Can you work these out from the model? Positions are in its coordinate system, mm. Face numbers are marked on the shaded views. Round coordinates to 2 decimals unless told otherwise and drop trailing zeros. Write each loop counter-clockwise with the first axis right and the second up, starting at its lowest first coordinate (ties: lowest second). Pieces come first, ordered by that corner, then holes. Notation, with made-up numbers: (42, -30) - (84, -30) arc R21 cw to (84, 1) - close; hole circle Ø2 at (-26.5, 62). An arc over 180 degrees is marked (long way). One line per item, written item: value. Start each with the question number.
(1) Thinking about a two-plate mould opening in Y: for the marked faces 1, 2 and 3, which applies, +Y half, -Y half, draft (parallel to the pull), parting line (faces both ways), or undercut?
(2) I want a section at D-D on x = 20. List the corners of the cut face in (y, z) for me.
(3) I want a section at C-C on y = -6. List the corners of the cut face in (x, z) for me.
(4) I'm going to push flat-ended pins straight in: pin 1 Ø1.1 at (y, z) = (-3, 8.5) entering from +X; pin 2 Ø0.6 at (x, y) = (26, -6.5) entering from -Z; pin 3 Ø1.1 at (x, y) = (13.5, 2.5) entering from -Z. Where does each tip first touch, or does it pass through?
(5) If I drill on L1, parallel to Y at x = 25.5, z = 19; L2, parallel to Y at x = 16.5, z = 11.75; L3, parallel to Y at x = 34, z = 23, over which ranges is the centre line in solid material (lowest first)? Write a range as from..to.
(6) I want a section at B-B on z = 17. List the corners of the cut face in (x, y) for me, plus the area to 3 significant figures.
(7) I want a section at A-A on z = 20.5. List the corners of the cut face in (x, y) for me.
from build123d import *

# Parameters (mm, degrees)
SKETCH1_W           = 3
SKETCH1_H           = 21.71695
SKETCH1_W_2         = 2.8
SKETCH1_H_2         = 4
SKETCH1_W_3         = 0.2
BOSS_EXTRUDE3_DEPTH = 1.36
BOSS_EXTRUDE4_START = -1.36
SKETCH1_7_W         = 3
SKETCH1_7_H         = 21.71695
SKETCH1_7_W_2       = 2.8
SKETCH1_7_H_2       = 4
SKETCH1_7_W_3       = 0.2
BOSS_EXTRUDE4_DEPTH = 2.2
BOSS_EXTRUDE5_START = -3.56
SKETCH1_8_W         = 3
SKETCH1_8_H         = 21.71695
BOSS_EXTRUDE5_DEPTH = 1.7
BOSS_EXTRUDE6_START = -5.26
SKETCH1_9_W         = 3
SKETCH1_9_H         = 21.71695
SKETCH1_9_W_2       = 2.8
SKETCH1_9_H_2       = 4
SKETCH1_9_W_3       = 0.2
BOSS_EXTRUDE6_DEPTH = 2
SKETCH2_W           = 43.56375
SKETCH2_H           = 3
BOSS_EXTRUDE7_DEPTH = 1.8
BOSS_EXTRUDE8_START = 1.8
SKETCH2_3_W         = 43.56375
SKETCH2_3_H         = 3
BOSS_EXTRUDE8_DEPTH = 1.8


with BuildPart() as part:
    # Sketch1 → Boss-Extrude3 (new body)
    with BuildSketch(Plane(origin=(0, 0, 0), x_dir=(1, 0, 0), z_dir=(0, 1, 0))):
        Polygon((2.8, -21.51695), (-0.2, -21.51695), (-3.2, -21.51695), (-3.2, -24.51695), (40.36375, -24.51695), (40.36375, -21.51695), align=None)
        with Locations((-1.7, -10.658475)):
            Rectangle(SKETCH1_W, SKETCH1_H)
        Polygon((0, 0), (0, -21.31695), (2.8, -21.31695), (2.8, -18.51695), (2.8, 0), align=None)
        Polygon((40.16375, 0), (2.8, 0), (2.8, -18.51695), (37.36375, -18.51695), (37.36375, -14.51695), (40.16375, -14.51695), align=None)
        Polygon((2.8, -18.51695), (2.8, -21.31695), (40.16375, -21.31695), (40.16375, -18.51695), (37.36375, -18.51695), align=None)
        with Locations((38.76375, -16.51695)):
            Rectangle(SKETCH1_W_2, SKETCH1_H_2)
        Polygon((43.36375, -14.51695), (40.36375, -14.51695), (40.36375, -18.51695), (40.36375, -21.51695), (40.36375, -24.51695), (43.36375, -24.51695), align=None)
        Polygon((2.8, -21.31695), (2.8, -21.51695), (40.36375, -21.51695), (40.36375, -18.51695), (40.16375, -18.51695), (40.16375, -21.31695), align=None)
        Polygon((40.36375, 0.2), (2.8, 0.2), (2.8, 0), (40.16375, 0), (40.16375, -14.51695), (40.36375, -14.51695), align=None)
        with Locations((40.26375, -16.51695)):
            Rectangle(SKETCH1_W_3, SKETCH1_H_2)
        Polygon((0, -21.31695), (-0.2, -21.31695), (-0.2, -21.51695), (2.8, -21.51695), (2.8, -21.31695), align=None)
        Polygon((2.8, 0.2), (-0.2, 0.2), (-0.2, -21.31695), (0, -21.31695), (0, 0), (2.8, 0), align=None)
    extrude(amount=-BOSS_EXTRUDE3_DEPTH)

    # Sketch1<7> → Boss-Extrude4 (add)
    with BuildSketch(Plane(origin=(0, 0, 0), x_dir=(1, 0, 0), z_dir=(0, 1, 0)).offset(BOSS_EXTRUDE4_START)):
        Polygon((0, 0), (0, -21.31695), (2.8, -21.31695), (2.8, -18.51695), (2.8, 0), align=None)
        with Locations((-1.7, -10.658475)):
            Rectangle(SKETCH1_7_W, SKETCH1_7_H)
        Polygon((2.8, 0.2), (-0.2, 0.2), (-0.2, -21.31695), (0, -21.31695), (0, 0), (2.8, 0), align=None)
        Polygon((0, -21.31695), (-0.2, -21.31695), (-0.2, -21.51695), (2.8, -21.51695), (2.8, -21.31695), align=None)
        Polygon((2.8, -21.51695), (-0.2, -21.51695), (-3.2, -21.51695), (-3.2, -24.51695), (40.36375, -24.51695), (40.36375, -21.51695), align=None)
        Polygon((2.8, -21.31695), (2.8, -21.51695), (40.36375, -21.51695), (40.36375, -18.51695), (40.16375, -18.51695), (40.16375, -21.31695), align=None)
        Polygon((2.8, -18.51695), (2.8, -21.31695), (40.16375, -21.31695), (40.16375, -18.51695), (37.36375, -18.51695), align=None)
        with Locations((38.76375, -16.51695)):
            Rectangle(SKETCH1_7_W_2, SKETCH1_7_H_2)
        Polygon((43.36375, -14.51695), (40.36375, -14.51695), (40.36375, -18.51695), (40.36375, -21.51695), (40.36375, -24.51695), (43.36375, -24.51695), align=None)
        with Locations((40.26375, -16.51695)):
            Rectangle(SKETCH1_7_W_3, SKETCH1_7_H_2)
    extrude(amount=-BOSS_EXTRUDE4_DEPTH)

    # Sketch1<8> → Boss-Extrude5 (add)
    with BuildSketch(Plane(origin=(0, 0, 0), x_dir=(1, 0, 0), z_dir=(0, 1, 0)).offset(BOSS_EXTRUDE5_START)):
        with Locations((-1.7, -10.658475)):
            Rectangle(SKETCH1_8_W, SKETCH1_8_H)
        Polygon((2.8, -21.51695), (-0.2, -21.51695), (-3.2, -21.51695), (-3.2, -24.51695), (40.36375, -24.51695), (40.36375, -21.51695), align=None)
        Polygon((43.36375, -14.51695), (40.36375, -14.51695), (40.36375, -18.51695), (40.36375, -21.51695), (40.36375, -24.51695), (43.36375, -24.51695), align=None)
    extrude(amount=-BOSS_EXTRUDE5_DEPTH)

    # Sketch1<9> → Boss-Extrude6 (add)
    with BuildSketch(Plane(origin=(0, 0, 0), x_dir=(1, 0, 0), z_dir=(0, 1, 0)).offset(BOSS_EXTRUDE6_START)):
        with Locations((-1.7, -10.658475)):
            Rectangle(SKETCH1_9_W, SKETCH1_9_H)
        Polygon((0, 0), (0, -21.31695), (2.8, -21.31695), (2.8, -18.51695), (2.8, 0), align=None)
        Polygon((2.8, -21.51695), (-0.2, -21.51695), (-3.2, -21.51695), (-3.2, -24.51695), (40.36375, -24.51695), (40.36375, -21.51695), align=None)
        Polygon((2.8, -18.51695), (2.8, -21.31695), (40.16375, -21.31695), (40.16375, -18.51695), (37.36375, -18.51695), align=None)
        Polygon((43.36375, -14.51695), (40.36375, -14.51695), (40.36375, -18.51695), (40.36375, -21.51695), (40.36375, -24.51695), (43.36375, -24.51695), align=None)
        with Locations((38.76375, -16.51695)):
            Rectangle(SKETCH1_9_W_2, SKETCH1_9_H_2)
        Polygon((2.8, -21.31695), (2.8, -21.51695), (40.36375, -21.51695), (40.36375, -18.51695), (40.16375, -18.51695), (40.16375, -21.31695), align=None)
        with Locations((40.26375, -16.51695)):
            Rectangle(SKETCH1_9_W_3, SKETCH1_9_H_2)
        Polygon((0, -21.31695), (-0.2, -21.31695), (-0.2, -21.51695), (2.8, -21.51695), (2.8, -21.31695), align=None)
        Polygon((2.8, 0.2), (-0.2, 0.2), (-0.2, -21.31695), (0, -21.31695), (0, 0), (2.8, 0), align=None)
    extrude(amount=-BOSS_EXTRUDE6_DEPTH)

    # Sketch2 → Boss-Extrude7 (add)
    with BuildSketch(Plane(origin=(0, 0, 0), x_dir=(1, 0, 0), z_dir=(0, 1, 0))):
        with Locations((18.581875, -9.21695)):
            Rectangle(SKETCH2_W, SKETCH2_H)
    extrude(amount=BOSS_EXTRUDE7_DEPTH)

    # Sketch2<3> → Boss-Extrude8 (add)
    with BuildSketch(Plane(origin=(0, 0, 0), x_dir=(1, 0, 0), z_dir=(0, 1, 0)).offset(BOSS_EXTRUDE8_START)):
        Polygon((40.36375, -10.71695), (-3.2, -10.71695), (-3.2, -24.51695), (40.36375, -24.51695), (40.36375, -14.51695), align=None)
        with Locations((18.581875, -9.21695)):
            Rectangle(SKETCH2_3_W, SKETCH2_3_H)
    extrude(amount=BOSS_EXTRUDE8_DEPTH)


solid = part.part
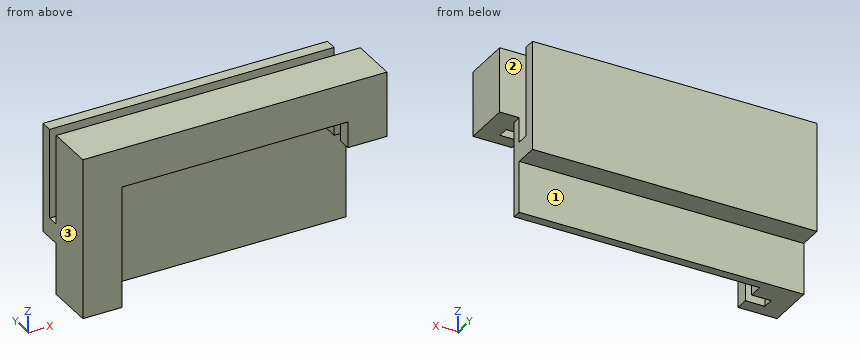
Established:
1. face 1: +Y half
1. face 2: undercut
1. face 3: draft
2. outline: (-7.26, 18.52) - (-5.26, 18.52) - (-5.26, 21.52) - (-3.56, 21.52) - (-3.56, 18.52) - (-1.36, 18.52) - (-1.36, -0.2) - (0, -0.2) - (0, 7.72) - (3.6, 7.72) - (3.6, 24.52) - (1.8, 24.52) - (1.8, 10.72) - (0, 10.72) - (0, 24.52) - (-7.26, 24.52) - close
3. outline: (-3.2, -0.2) - (2.8, -0.2) - (2.8, 18.52) - (37.36, 18.52) - (37.36, 14.52) - (43.36, 14.52) - (43.36, 24.52) - (-3.2, 24.52) - close
4. pin 1: x = 2.8
4. pin 2: z = 18.52
4. pin 3: z = 7.72
5. L1: -7.26..-5.26, -3.56..0, 1.8..3.6
5. L2: -1.36..0, 1.8..3.6
5. L3: -7.26..0, 1.8..3.6
6. outline: (-3.2, -7.26) - (2.8, -7.26) - (2.8, -5.26) - (-0.2, -5.26) - (-0.2, -3.56) - (2.8, -3.56) - (2.8, -1.36) - (37.36, -1.36) - (37.36, -3.56) - (40.36, -3.56) - (40.36, -5.26) - (37.36, -5.26) - (37.36, -7.26) - (43.36, -7.26) - (43.36, 0) - (-3.2, 0) - close; (-3.2, 1.8) - (40.36, 1.8) - (40.36, 3.6) - (-3.2, 3.6) - close
6. area: 202 mm2
7. outline: (-3.2, -7.26) - (43.36, -7.26) - (43.36, 0) - (-3.2, 0) - close; (-3.2, 1.8) - (40.36, 1.8) - (40.36, 3.6) - (-3.2, 3.6) - close; hole (-0.2, -5.26) - (40.36, -5.26) - (40.36, -3.56) - (-0.2, -3.56) - close
